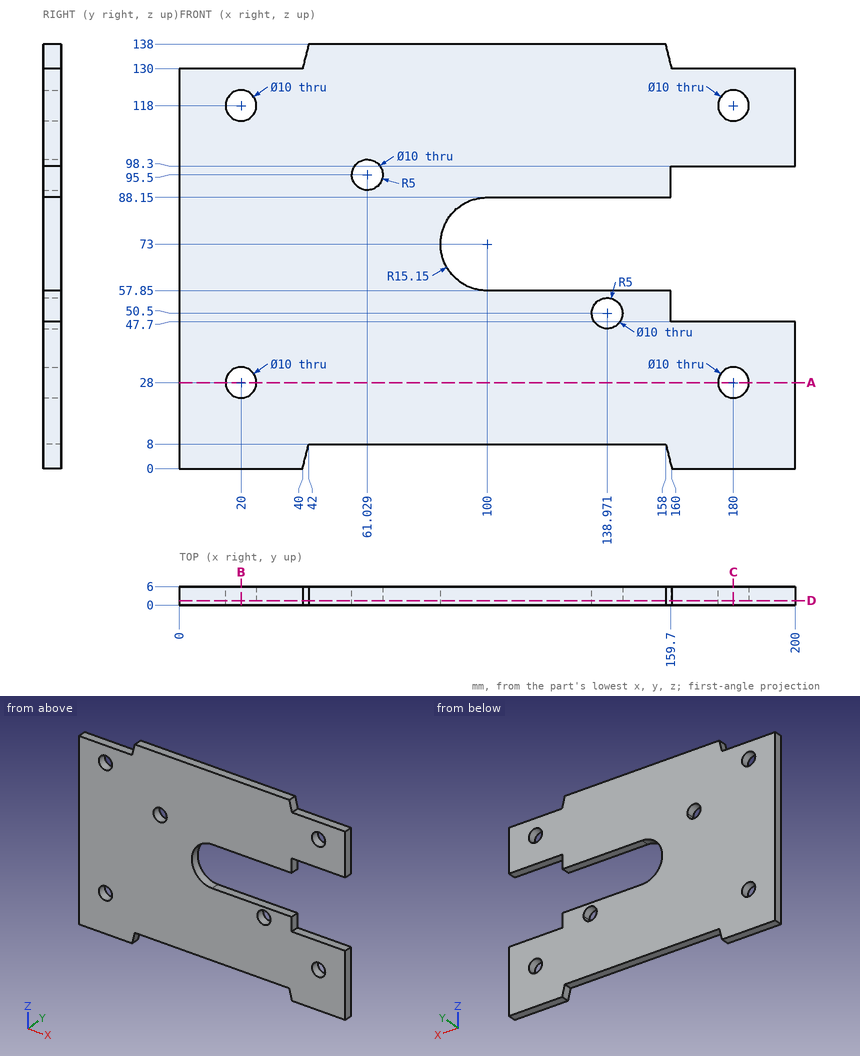
Part print with two shaded views. Sizes in mm from the minimum x, y, z corner. Coordinates: 2 decimals unless noted, no trailing zeros. Write each loop counter-clockwise with the first axis right and the second up, starting at its lowest first coordinate (ties: lowest second). Pieces come first, ordered by that corner, then holes.
(1) Cut at C-C on x = 180. List the corners of the cut face in (y, z).
(2) Pin check, flat tips, straight feed: pin 1 Ø1.8 at (x, y) = (176, 2) entering from +Z; pin 2 Ø3 at (x, y) = (127.5, 4.5) entering from -Z. Stop position of each tip, or through.
(3) Cut at B-B on x = 20. List the corners of the cut face in (y, z).
(4) Cut at A-A on z = 28. List the corners of the cut face in (x, y).
(5) Cut at D-D on y = 1.45. State how many separate pieces and enclosed holes the cut face has, and give its area (3 significant figures).
(6) Drill centre lines: line 1 (Z direction, x = 20, y = 2.6); line 2 (Z direction, x = 138.5, y = 3); line 3 (Z direction, x = 180, y = 4.65). Where is each one in solid material? Low to high.
Working result:
1. outline: (0, 0) - (6, 0) - (6, 23) - (0, 23) - close; (0, 33) - (6, 33) - (6, 47.7) - (0, 47.7) - close; (0, 98.3) - (6, 98.3) - (6, 113) - (0, 113) - close; (0, 123) - (6, 123) - (6, 130) - (0, 130) - close
2. pin 1: stops at z = 130
2. pin 2: stops at z = 8
3. outline: (0, 0) - (6, 0) - (6, 23) - (0, 23) - close; (0, 33) - (6, 33) - (6, 113) - (0, 113) - close; (0, 123) - (6, 123) - (6, 130) - (0, 130) - close
4. outline: (0, 0) - (15, 0) - (15, 6) - (0, 6) - close; (25, 0) - (175, 0) - (175, 6) - (25, 6) - close; (185, 0) - (200, 0) - (200, 6) - (185, 6) - close
5. separate pieces: 1
5. enclosed holes: 6
5. area: 21,300 mm2
6. line 1: z = 0 to 23, 33 to 113, 123 to 130
6. line 2: z = 8 to 45.52, 55.48 to 57.85, 88.15 to 138
6. line 3: z = 0 to 23, 33 to 47.7, 98.3 to 113, 123 to 130
